from build123d import *

# Parameters (mm, degrees)
F0_W      = 65
F0_H      = 35
F0_W_2    = 57
F0_H_2    = 27
F1_DEPTH  = 784
F2_W      = 100
F2_H      = 150
F3_DEPTH  = 16
F5_D      = 18
F6_W      = 535
F6_H      = 150
F7_DEPTH  = 10
F9_D      = 18
F10_W     = 65
F10_H     = 35
F11_DEPTH = 5


with BuildPart() as f1:
    # F0 (on Front) → F1 (new body)
    with BuildSketch(Plane.XZ):
        Rectangle(F0_W, F0_H)
        Rectangle(F0_W_2, F0_H_2, mode=Mode.SUBTRACT)
    extrude(amount=F1_DEPTH)

    # F2 (on face) → F3 (join)
    with BuildSketch(Plane.XZ.offset(784)):
        Rectangle(F2_W, F2_H)
    extrude(amount=F3_DEPTH)

    # F5 (through all)
    with Locations(Plane.XZ.offset(800)):
        with Locations((0, 50), (0, -50)):
            Hole(F5_D / 2)

    # F6 (on face) → F7 (join)
    with BuildSketch(Plane.YZ.offset(32.5)):
        with Locations((-365.592288, 0.218023)):
            Rectangle(F6_W, F6_H)
    extrude(amount=F7_DEPTH)

    # F9 (through all)
    with Locations(Plane.YZ.offset(42.5)):
        with Locations((-148.092288, 46.218023), (-148.092288, -46.781977), (-583.092288, -46.781977), (-583.092288, 46.218023)):
            Hole(F9_D / 2)

    # F10 (on face) → F11 (join)
    with BuildSketch(Plane(origin=(0, 0, 0), x_dir=(-1, 0, 0), z_dir=(0, 1, 0))):
        Rectangle(F10_W, F10_H)
    extrude(amount=F11_DEPTH)


solid = f1.part
Part model, mm, in its own coordinate system. A direction names the side the tool comes from. Give positions to 0.01 mm unless a question says otherwise; leave off trailing zeros. Loops run counter-clockwise (first coordinate to the right, second up) from the corner with the lowest first, then second, coordinate; pieces in that order, holes last.
(1) Pin check, flat tips, straight feed: pin 1 (16 mm diameter, centred on y = -583.09, z = 46.22, fed in from +X); pin 2 (1.5 mm diameter, centred on y = -500.5, z = 15, fed in from -X); pin 3 (1 mm diameter, centred on y = -356, z = -50.5, fed in from -X); pin 4 (8 mm diameter, centred on x = 35.5, z = -35, fed in from +Y). Stop position of each tip, or through.
Return value:
pin 1: passes through
pin 2: stops at x = -32.5
pin 3: stops at x = 32.5
pin 4: stops at y = -98.09
(2) Pull direction Z, two halves, no side cores. Call faces 4 (the flat face through (-32.5, -395, 0)), 5 (the cylindrical face through (-4.84, -791.89, -42.41)), 6 (the flat face through (-1, -792, -75)): pulls with the +Z half, pulls with the -Z half, needs draft (parallel to the pull), parting line crosses it, or undercut.
Return value:
face 4: needs draft
face 5: undercut
face 6: pulls with the -Z half
(3) Drill centre lines: line 1 along Z through (x, y) = (0, -789); line 2 along Z through (x, y) = (-13, -563); line 3 along X through (y, z) = (-689.5, 0). Where is each one in solid material? Low to high.
Return value:
line 1: z = -75 to -59, -41 to 41, 59 to 75
line 2: z = -17.5 to -13.5, 13.5 to 17.5
line 3: x = -32.5 to -28.5, 28.5 to 32.5
(4) Band-saw the part on B-B (y = -420). Write the cut outline in (x, z), and give its area (3 significant figures).
Return value:
outline: (-32.5, -17.5) - (32.5, -17.5) - (32.5, -74.78) - (42.5, -74.78) - (42.5, 75.22) - (32.5, 75.22) - (32.5, 17.5) - (-32.5, 17.5) - close; hole (-28.5, -13.5) - (28.5, -13.5) - (28.5, 13.5) - (-28.5, 13.5) - close
area: 2,240 mm2
(5) Band-saw the part on C-C (y = -74). Write the cut outline in (x, z).
Return value:
outline: (-32.5, -17.5) - (32.5, -17.5) - (32.5, 17.5) - (-32.5, 17.5) - close; hole (-28.5, -13.5) - (28.5, -13.5) - (28.5, 13.5) - (-28.5, 13.5) - close
(6) Band-saw the part on A-A (x = 0). Write the cut outline in (y, z).
Return value:
outline: (-800, -75) - (-784, -75) - (-784, -59) - (-800, -59) - close; (-800, -41) - (-784, -41) - (-784, -17.5) - (5, -17.5) - (5, 17.5) - (-784, 17.5) - (-784, 41) - (-800, 41) - close; (-800, 59) - (-784, 59) - (-784, 75) - (-800, 75) - close; hole (-784, -13.5) - (0, -13.5) - (0, 13.5) - (-784, 13.5) - close
(7) 3-axis set-ups, long thin cutter, end or side, ignore diameter. For faces 1 (the flat face through (0, -395, 17.5)), 2 (the flat face through (-28.5, -387, 0)), 3 (the flat face through (32.5, -47, 0)): which of +Z, -Z, +X, -X, +Y, -Y reach the whole face in a straight line?
Return value:
face 1: +Z, -X, +Y
face 2: none
face 3: +Z, -Z, +X, +Y
